Check sheet for the modelled part. Datum: model origin and axes. Units: mm. Give positions to 0.01 mm unless a question says otherwise; leave off trailing zeros. Write each loop counter-clockwise with the first axis right and the second up, starting at its lowest first coordinate (ties: lowest second). Pieces come first, ordered by that corner, then holes. Notation, with made-up numbers: (55.5, -37.75) -> (78.5, -37.75) arc R24 ccw to (78.5, -1.75) -> close; hole circle Ø10 at (-38, 47.25). An arc over 180 degrees is marked (long way). Answer as a JSON object with one key per item and string values.
from build123d import *

# Parameters (mm, degrees)
SKETCH1_R           = 8
SKETCH1_R_2         = 1.25
BOSS_EXTRUDE1_DEPTH = 3


with BuildPart() as part:
    # Sketch1 → Boss-Extrude1 (new body)
    with BuildSketch(Plane(origin=(0, 0, 0), x_dir=(1, 0, 0), z_dir=(0, 1, 0))):
        Polygon((-42, 45), (42, 45), (76, 67), (106, 67), (125, 45), (125, -18), (108, -33), (78, -33), (60, -45), (-60, -45), (-78, -33), (-108, -33), (-125, -18), (-125, 45), (-106, 67), (-76, 67), align=None)
        with Locations(Location((-90, -3, 0), (0, 0, 270))):
            Circle(SKETCH1_R, mode=Mode.SUBTRACT)
        with Locations(Location((90, -3, 0), (0, 0, 270))):
            Circle(SKETCH1_R, mode=Mode.SUBTRACT)
        with Locations(Location((-72.7, -7, 0), (0, 0, 270))):
            Circle(SKETCH1_R_2, mode=Mode.SUBTRACT)
        with Locations(Location((-107.3, -7, 0), (0, 0, 270))):
            Circle(SKETCH1_R_2, mode=Mode.SUBTRACT)
        with Locations(Location((72.7, -7, 0), (0, 0, 270))):
            Circle(SKETCH1_R_2, mode=Mode.SUBTRACT)
        with Locations(Location((107.3, -7, 0), (0, 0, 270))):
            Circle(SKETCH1_R_2, mode=Mode.SUBTRACT)
    extrude(amount=BOSS_EXTRUDE1_DEPTH)


solid = part.part
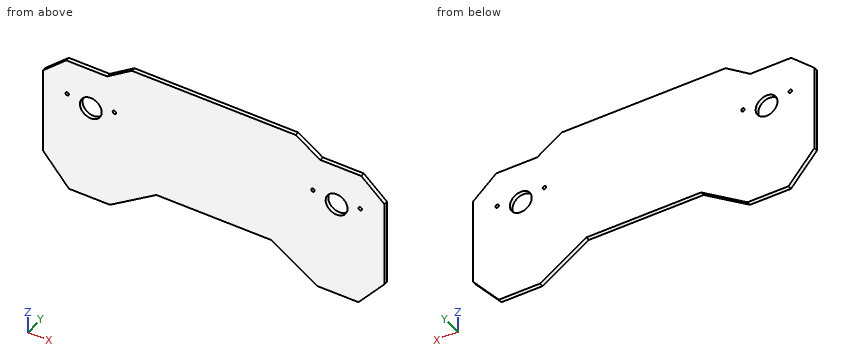
1. Go/stop test with flat-tipped pins: P1, Ø0.9, axis at x = -90.5, y = 1, coming from the +Z side; P2, Ø1, axis at x = -69, y = 1, coming from the -Z side. Record where each tip stops, or that it passes through.
Determined:
{"P1": "z = 33", "P2": "z = -62.79"}
2. Sectioned sample at B-B, the plane z = 2. Enter the section's corners in (x, y), plus the area to 3 significant figures.
Determined:
{"outline": "(-125, 0) -> (-97.94, 0) -> (-97.94, 3) -> (-125, 3) -> close; (-82.06, 0) -> (82.06, 0) -> (82.06, 3) -> (-82.06, 3) -> close; (97.94, 0) -> (125, 0) -> (125, 3) -> (97.94, 3) -> close", "area": "655 mm^2"}
3. Sectioned sample at D-D, the plane z = -53.5. Enter the section's corners in (x, y), plus the area to 3 significant figures.
Determined:
{"outline": "(-117.66, 0) -> (-55.14, 0) -> (-55.14, 3) -> (-117.66, 3) -> close; (55.14, 0) -> (117.66, 0) -> (117.66, 3) -> (55.14, 3) -> close", "area": "375 mm^2"}
4. Sectioned sample at A-A, the plane x = 90. Enter the section's corners in (y, z), plus the area to 3 significant figures.
Determined:
{"outline": "(0, -67) -> (3, -67) -> (3, -5) -> (0, -5) -> close; (0, 11) -> (3, 11) -> (3, 33) -> (0, 33) -> close", "area": "252 mm^2"}
5. Scan lines: L1, parallel to X at y = 2, z = 3; L2, parallel to Z at x = 72, y = 0.85; L3, parallel to Z at x = -72.7, y = 1.6. Record each from-to range of solid material in increasing order. Write a range as [from, to].
Determined:
{"L1": "[-125, -98], [-82, 82], [98, 125]", "L2": "[-64.41, 5.96], [8.04, 37]", "L3": "[-64.86, 5.75], [8.25, 36.53]"}
6. Sectioned sample at C-C, the plane y = 2. Enter the section's corners in (x, z), plus the area to 3 significant figures.
Determined:
{"outline": "(-125, -45) -> (-106, -67) -> (-76, -67) -> (-42, -45) -> (42, -45) -> (76, -67) -> (106, -67) -> (125, -45) -> (125, 18) -> (108, 33) -> (78, 33) -> (60, 45) -> (-60, 45) -> (-78, 33) -> (-108, 33) -> (-125, 18) -> close; hole circle Ø2.5 at (-107.3, 7); hole circle Ø16 at (-90, 3); hole circle Ø2.5 at (-72.7, 7); hole circle Ø2.5 at (72.7, 7); hole circle Ø16 at (90, 3); hole circle Ø2.5 at (107.3, 7)", "area": "23,000 mm^2"}
